Check sheet for the modelled part. Datum: model origin and axes. Units: mm. A direction names the side the tool comes from. Give positions to 0.01 mm unless a question says otherwise; leave off trailing zeros. Loops run counter-clockwise (first coordinate to the right, second up) from the corner with the lowest first, then second, coordinate; pieces in that order, holes last. Notation, with made-up numbers: (-34, 3.25) -> (-19, 3.25) arc R18 cw to (-19, 7.25) -> close; hole circle Ø2 at (12.25, 29). An arc over 180 degrees is marked (long way). Write each question's results on one line, items separated by ' | '. Start each with the question number.
Item 1: Cross-section at C-C on x = 1.1. Enter the section's corners in (y, z).
Item 2: Access from +Z, -Z, +X, -X, +Y, -Y to the whole of each face (thin tool, end or side, straight path). Record for faces 1 (the face through (5, -7.7, -15.5)), 2 (the face through (3.99, 20.03, 6.31)).
Item 3: Cross-section at D-D on y = -9.5. Enter the section's corners in (x, z), then the cut area to 3 significant figures.
Item 4: Cross-section at A-A on y = 0. Enter the section's corners in (x, z).
Item 5: Mould release check, pull along Z, two halves, no side actions. Record for faces 3 (the face through (3, 9, 20)), 4 (the face through (1.48, -29.97, 1.32)), 5 (the face through (1.521, -22.804, -0.488)), 6 (the face through (1.521, -0.488, 22.804)): pulls with the +Z half, pulls with the -Z half, needs draft (parallel to the pull), parting line crosses it, or undercut.
Item 6: Scan lines: line 1 along Z through (x, y) = (0.7, 0); line 2 along Z through (x, y) = (2.1, 2); line 3 along X through (y, z) = (-23, -14.5). Record each from-to range of solid material in increasing order.
Item 7: Gauge pin test, flat ends, axial feed: pin 1 Ø10 at (y, z) = (-15, 3) entering from +X; pin 2 Ø4 at (y, z) = (-19.5, -14.5) entering from +X; pin 3 Ø1.5 at (x, y) = (4, -7.5) entering from -Z; pin 4 Ø3 at (x, z) = (3.5, -6) entering from -Y. Record the tip position at first contact, or that the pin passes through.
Item 8: Cross-section at B-B on z = -1.5. Enter the section's corners in (x, y).
from build123d import *

# Parameters (mm, degrees)
M4_CLEARANCE_HOLE1_D     = 4.5
M4_CLEARANCE_HOLE1_DEPTH = 3.001
CIRPATTERN1_COUNT        = 4


with BuildPart() as part:
    # Sketch1 → Revolve1 (revolve)
    with BuildSketch(Plane.XY):
        Polygon((0, 17), (5, 17), (5, 21), (3, 21), (3, 30), (0, 30), align=None)
    revolve(axis=Axis((0, 0, 0), (1, 0, 0)))

    # M4 Clearance Hole1
    with Locations(Plane.ZY):
        with Locations((0, 25)):
            m4_clearance_hole1 = Hole(M4_CLEARANCE_HOLE1_D / 2, depth=M4_CLEARANCE_HOLE1_DEPTH)

    # CirPattern1: M4 Clearance Hole1 ×4 about axis
    cirpattern1_axis = Axis((0, 0, 0), (1, 0, 0))
    for i in range(1, CIRPATTERN1_COUNT):
        add(m4_clearance_hole1.rotate(cirpattern1_axis, i * 360 / CIRPATTERN1_COUNT), mode=Mode.SUBTRACT)


solid = part.part
Answer sheet:
1) outline: circle Ø60 at (0, 0); hole circle Ø4.5 at (-25, 0); hole circle Ø34 at (0, 0); hole circle Ø4.5 at (0, -25); hole circle Ø4.5 at (0, 25); hole circle Ø4.5 at (25, 0)
2) face 1: +Z, -Z, +X, +Y, -Y | face 2: +X
3) outline: (0, -28.46) -> (3, -28.46) -> (3, -18.73) -> (5, -18.73) -> (5, -14.1) -> (0, -14.1) -> close; (0, 14.1) -> (5, 14.1) -> (5, 18.73) -> (3, 18.73) -> (3, 28.46) -> (0, 28.46) -> close | area: 105 mm²
4) outline: (0, -30) -> (3, -30) -> (3, -27.25) -> (0, -27.25) -> close; (0, -22.75) -> (3, -22.75) -> (3, -21) -> (5, -21) -> (5, -17) -> (0, -17) -> close; (0, 17) -> (5, 17) -> (5, 21) -> (3, 21) -> (3, 22.75) -> (0, 22.75) -> close; (0, 27.25) -> (3, 27.25) -> (3, 30) -> (0, 30) -> close
5) face 3: needs draft | face 4: parting line crosses it | face 5: undercut | face 6: undercut
6) line 1: z = -30 to -27.25, -22.75 to -17, 17 to 22.75, 27.25 to 30 | line 2: z = -29.93 to -26.03, -23.97 to -16.88, 16.88 to 23.97, 26.03 to 29.93 | line 3: x = 0 to 3
7) pin 1: stops at x = 5 | pin 2: stops at x = 3 | pin 3: stops at z = -19.89 | pin 4: stops at y = -29.65
8) outline: (0, -29.96) -> (3, -29.96) -> (3, -26.68) -> (0, -26.68) -> close; (0, -23.32) -> (3, -23.32) -> (3, -20.95) -> (5, -20.95) -> (5, -16.93) -> (0, -16.93) -> close; (0, 16.93) -> (5, 16.93) -> (5, 20.95) -> (3, 20.95) -> (3, 23.32) -> (0, 23.32) -> close; (0, 26.68) -> (3, 26.68) -> (3, 29.96) -> (0, 29.96) -> close
